Geometry check sheet. Reference: the model listing, model coordinates, mm. Face numbers are marked on the shaded views. A direction names the side the tool comes from. Round coordinates to 2 decimals unless told otherwise and drop trailing zeros. Write each loop counter-clockwise with the first axis right and the second up, starting at its lowest first coordinate (ties: lowest second). Pieces come first, ordered by that corner, then holes.
from build123d import *

# Parameters (mm, degrees)
F0_R     = 1
F1_DEPTH = 3.5
F2_DEPTH = 2
F3_DEPTH = 2


with BuildPart() as f1:
    # F0 (on Top) → F1 (new body)
    with BuildSketch(Plane.XY):
        with Locations((-2.3999998812, 1.8953582125)):
            Circle(F0_R)
    extrude(amount=F1_DEPTH)



with BuildPart() as f1b:
    # F0 (on Top) → F1, piece 2 (new body)
    with BuildSketch(Plane.XY):
        with Locations((1.6000001188, 1.8953582125)):
            Circle(F0_R)
    extrude(amount=F1_DEPTH)


with BuildPart() as f1c:
    # F0 (on Top) → F1, piece 3 (new body)
    with BuildSketch(Plane.XY):
        with Locations((1.6000001188, -2.0999999251)):
            Circle(F0_R)
    extrude(amount=F1_DEPTH)


with BuildPart() as f1d:
    # F0 (on Top) → F1, piece 4 (new body)
    with BuildSketch(Plane.XY):
        with Locations((-2.3999998812, -2.0999999251)):
            Circle(F0_R)
    extrude(amount=F1_DEPTH)


with BuildPart() as f1_1:
    add(f1.part)

    add(f1d.part)  # F2 merges F1d
    # F0 (on Top) → F2 (join)
    with BuildSketch(Plane.XY):
        with BuildLine():
            ThreePointArc((-2.4963240114, -0.1023208563), (-3.7797374902, -3.5478687487), (-0.3999998812, -2.0999999251))
            ThreePointArc((-0.3999998812, -2.0999999251), (-0.9521310576, -0.7202623161), (-2.3036757509, -0.1023208563))
            ThreePointArc((-2.3036757509, -0.1023208563), (-2.3999998812, -0.1046417875), (-2.4963240114, -0.1023208563))
        make_face()
        with Locations((-2.3999998812, -2.0999999251)):
            Circle(F0_R, mode=Mode.SUBTRACT)
        with BuildLine():
            ThreePointArc((-2.4963240114, -0.1023208563), (-2.3999998812, -0.1046417875), (-2.3036757509, -0.1023208563))
            ThreePointArc((-2.3036757509, -0.1023208563), (-2.3999998812, -0.0999999251), (-2.4963240114, -0.1023208563))
        make_face()
        with BuildLine():
            ThreePointArc((-2.4963240114, -0.1023208563), (-2.3999998812, -0.0999999251), (-2.3036757509, -0.1023208563))
            ThreePointArc((-2.3036757509, -0.1023208563), (-0.9521310576, 0.5156206035), (-0.3999998812, 1.8953582125))
            ThreePointArc((-0.3999998812, 1.8953582125), (-3.7797374902, 3.343227036), (-2.4963240114, -0.1023208563))
        make_face()
        with Locations((-2.3999998812, 1.8953582125)):
            Circle(F0_R, mode=Mode.SUBTRACT)
    extrude(amount=F2_DEPTH)


    add(f1b.part)  # F2#2 merges F1b

    add(f1c.part)  # F2#2 merges F1c
    # F0 (on Top) → F2, piece 2 (join)
    with BuildSketch(Plane.XY):
        with BuildLine():
            ThreePointArc((1.5036759886, -0.1023208563), (0.1521312953, -0.7202623161), (-0.3999998812, -2.0999999251))
            ThreePointArc((-0.3999998812, -2.0999999251), (1.6000001188, -4.0999999251), (3.6000001188, -2.0999999251))
            ThreePointArc((3.6000001188, -2.0999999251), (3.0478689424, -0.7202623161), (1.6963242491, -0.1023208563))
            ThreePointArc((1.6963242491, -0.1023208563), (1.6000001188, -0.1046417875), (1.5036759886, -0.1023208563))
        make_face()
        with Locations((1.6000001188, -2.0999999251)):
            Circle(F0_R, mode=Mode.SUBTRACT)
        with BuildLine():
            ThreePointArc((-0.3999998812, 1.8953582125), (0.1521312953, 0.5156206035), (1.5036759886, -0.1023208563))
            ThreePointArc((1.5036759886, -0.1023208563), (1.6000001188, -0.0999999251), (1.6963242491, -0.1023208563))
            ThreePointArc((1.6963242491, -0.1023208563), (3.0478689424, 0.5156206035), (3.6000001188, 1.8953582125))
            ThreePointArc((3.6000001188, 1.8953582125), (1.6000001188, 3.8953582125), (-0.3999998812, 1.8953582125))
        make_face()
        with Locations((1.6000001188, 1.8953582125)):
            Circle(F0_R, mode=Mode.SUBTRACT)
        with BuildLine():
            ThreePointArc((1.6963242491, -0.1023208563), (1.6000001188, -0.0999999251), (1.5036759886, -0.1023208563))
            ThreePointArc((1.5036759886, -0.1023208563), (1.6000001188, -0.1046417875), (1.6963242491, -0.1023208563))
        make_face()
    extrude(amount=F2_DEPTH)

    # F0 (on Top) → F3 (join)
    with BuildSketch(Plane.XY):
        with BuildLine():
            ThreePointArc((-2.3036757509, -0.1023208563), (-0.9521310576, -0.7202623161), (-0.3999998812, -2.0999999251))
            ThreePointArc((-0.3999998812, -2.0999999251), (0.1521312953, -0.7202623161), (1.5036759886, -0.1023208563))
            ThreePointArc((1.5036759886, -0.1023208563), (0.1521312953, 0.5156206035), (-0.3999998812, 1.8953582125))
            ThreePointArc((-0.3999998812, 1.8953582125), (-0.9521310576, 0.5156206035), (-2.3036757509, -0.1023208563))
        make_face()
    extrude(amount=F3_DEPTH)


solid = f1_1.part
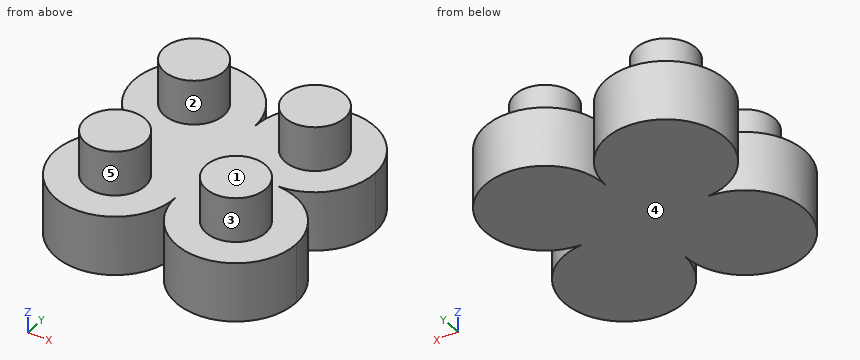
1. Scan lines: line 1 along Z through (x, y) = (2, -1); line 2 along X through (y, z) = (-1.5, 2.7); line 3 along Y through (x, z) = (-1.75, 2.05). Record each from-to range of solid material in increasing order.
2. Depth check by flat-ended pin: pin 1 Ø1.5 at (x, z) = (1, 2) entering from +Y; pin 2 Ø1.5 at (x, y) = (0, -3) entering from +Z. Enter the tip coordinate at first touch or a pass-through.
3. Access from +Z, -Z, +X, -X, +Y, -Y to the whole of each face (thin tool, end or side, straight path). Record for the marked faces 4 and 5.
4. Section check D-D (z = 2.9). Record the cut outline in (x, y), plus the area to 3 significant figures.
5. Section check C-C (x = 3.25). Record the cut outline in (y, z).
6. Release check for a two-part mould opening along Y. For the marked faces 1, 2 and 3 record: +Y half, -Y half, draft (parallel to the pull), parting line (faces both ways), or undercut.
7. Section check B-B (y = -2.25). Record the cut outline in (x, z), plus the area to 3 significant figures.
8. Section check A-A (x = 1.6). Record the cut outline in (y, z), plus the area to 3 significant figures.
Results below:
1. line 1: z = 0 to 2
1. line 2: x = -3.2 to -1.6, 0.8 to 2.4
1. line 3: y = -2.86 to -1.34, 1.14 to 2.66
2. pin 1: stops at y = 3.9
2. pin 2: stops at z = 2
3. face 4: -Z, +X, -X, +Y, -Y
3. face 5: +Z
4. outline: circle Ø2 at (-2.4, -2.1); circle Ø2 at (-2.4, 1.9); circle Ø2 at (1.6, -2.1); circle Ø2 at (1.6, 1.9)
4. area: 12.6 mm2
5. outline: (-3.23, 0) - (-0.97, 0) - (-0.97, 2) - (-3.23, 2) - close; (0.77, 0) - (3.03, 0) - (3.03, 2) - (0.77, 2) - close
6. face 1: draft
6. face 2: undercut
6. face 3: undercut
7. outline: (-4.39, 0) - (-0.41, 0) - (-0.41, 2) - (-1.41, 2) - (-1.41, 3.5) - (-3.39, 3.5) - (-3.39, 2) - (-4.39, 2) - close; (-0.39, 0) - (3.59, 0) - (3.59, 2) - (2.59, 2) - (2.59, 3.5) - (0.61, 3.5) - (0.61, 2) - (-0.39, 2) - close
7. area: 21.9 mm2
8. outline: (-4.1, 0) - (3.9, 0) - (3.9, 2) - (2.9, 2) - (2.9, 3.5) - (0.9, 3.5) - (0.9, 2) - (-1.1, 2) - (-1.1, 3.5) - (-3.1, 3.5) - (-3.1, 2) - (-4.1, 2) - close
8. area: 22.0 mm2
